```python
from build123d import *

# Parameters (mm, degrees)
SKETCH_1_R               = 15
SKETCH_1_R_2             = 2.3
SKETCH_1_R_3             = 1.1
EXTRUDE_1_DEPTH          = 7
CUT_EXTRUDE_1_DEPTH      = 10
CUT_EXTRUDE_1_DEPTH_BACK = 2
SKETCH_2_R               = 2.1
SKETCH_10_R              = 10
CUT_EXTRUDE_7_DEPTH      = 1.6
SKETCH_9_R               = 4.2
CUT_EXTRUDE_5_DEPTH      = 22.889723616
SKETCH_11_R              = 26.7
SKETCH_11_R_2            = 1.7
EXTRUDE_2_DEPTH          = 5.5
SKETCH_13_R              = 3
CUT_EXTRUDE_9_DEPTH      = 2.5
CUT_EXTRUDE_START        = -8
SKETCH_14_R              = 2.1
CUT_EXTRUDE_10_DEPTH     = 8


with BuildPart() as part:
    # 스케치1 → 보스-돌출1 (new body)
    with BuildSketch(Plane.XY):
        Circle(SKETCH_1_R)
        Circle(SKETCH_1_R_2, mode=Mode.SUBTRACT)
        with Locations((0, 8)):
            Circle(SKETCH_1_R_3, mode=Mode.SUBTRACT)
        with Locations((8, 0)):
            Circle(SKETCH_1_R_3, mode=Mode.SUBTRACT)
        with Locations((0, -8)):
            Circle(SKETCH_1_R_3, mode=Mode.SUBTRACT)
        with Locations((-8, 0)):
            Circle(SKETCH_1_R_3, mode=Mode.SUBTRACT)
    extrude(amount=EXTRUDE_1_DEPTH)

    # 스케치2 → 컷-돌출1 (cut, two sides: drawn at the far end of the back side and taken through both)
    with BuildSketch(Plane.XY.offset(7).offset(-CUT_EXTRUDE_1_DEPTH_BACK)):
        with Locations((0, 8)):
            Circle(SKETCH_2_R)
        with Locations((8, 0)):
            Circle(SKETCH_2_R)
        with Locations((0, -8)):
            Circle(SKETCH_2_R)
        with Locations((-8, 0)):
            Circle(SKETCH_2_R)
    extrude(amount=CUT_EXTRUDE_1_DEPTH + CUT_EXTRUDE_1_DEPTH_BACK, mode=Mode.SUBTRACT)

    # 스케치10 → 컷-돌출7 (cut)
    with BuildSketch(Plane(origin=(0, 0, 0), x_dir=(-1, 0, 0), z_dir=(0, 0, -1))):
        Circle(SKETCH_10_R)
    extrude(amount=-CUT_EXTRUDE_7_DEPTH, mode=Mode.SUBTRACT)

    # 스케치9 → 컷-돌출5 (cut, through all)
    with BuildSketch(Plane(origin=(0, 0, 1.6), x_dir=(-1, 0, 0), z_dir=(0, 0, -1))):
        Circle(SKETCH_9_R)
    extrude(amount=-CUT_EXTRUDE_5_DEPTH, mode=Mode.SUBTRACT)

    # 스케치11 → 보스-돌출2 (add)
    with BuildSketch(Plane.XY.offset(7)):
        Circle(SKETCH_11_R)
        with Locations((-11.254716834, 16.073401413)):
            Circle(SKETCH_11_R_2, mode=Mode.SUBTRACT)
        with Locations((-16.073401413, 11.254716834)):
            Circle(SKETCH_11_R_2, mode=Mode.SUBTRACT)
        with Locations((19.547332366, 1.710169984)):
            Circle(SKETCH_11_R_2, mode=Mode.SUBTRACT)
        with Locations((17.783571397, 8.292615532)):
            Circle(SKETCH_11_R_2, mode=Mode.SUBTRACT)
        with Locations((-8.292615532, -17.783571397)):
            Circle(SKETCH_11_R_2, mode=Mode.SUBTRACT)
        with Locations((-1.710169984, -19.547332366)):
            Circle(SKETCH_11_R_2, mode=Mode.SUBTRACT)
    extrude(amount=EXTRUDE_2_DEPTH)

    # 스케치13 → 컷-돌출9 (cut)
    with BuildSketch(Plane(origin=(0, 0, 7), x_dir=(-1, 0, 0), z_dir=(0, 0, -1))):
        with Locations((-17.783571397, 8.292615532)):
            Circle(SKETCH_13_R)
        with Locations((-19.547332366, 1.710169984)):
            Circle(SKETCH_13_R)
        with Locations((11.254716834, 16.073401413)):
            Circle(SKETCH_13_R)
        with Locations((16.073401413, 11.254716834)):
            Circle(SKETCH_13_R)
        with Locations((1.710169984, -19.547332366)):
            Circle(SKETCH_13_R)
        with Locations((8.292615532, -17.783571397)):
            Circle(SKETCH_13_R)
    extrude(amount=-CUT_EXTRUDE_9_DEPTH, mode=Mode.SUBTRACT)

    # 스케치14 → 컷-돌출10 (cut)
    with BuildSketch(Plane(origin=(0, 0, 7), x_dir=(-1, 0, 0), z_dir=(0, 0, -1)).offset(CUT_EXTRUDE_START)):
        with Locations(Location((8, 0, 0), (0, 0, 180))):
            Circle(SKETCH_14_R)
        with Locations(Location((0, -8, 0), (0, 0, 180))):
            Circle(SKETCH_14_R)
        with Locations(Location((-8, 0, 0), (0, 0, 180))):
            Circle(SKETCH_14_R)
        with Locations(Location((0, 8, 0), (0, 0, 180))):
            Circle(SKETCH_14_R)
    extrude(amount=CUT_EXTRUDE_10_DEPTH, mode=Mode.SUBTRACT)


solid = part.part
```
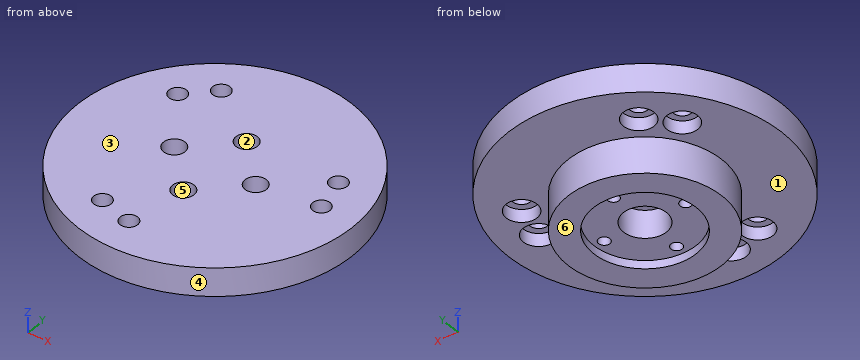
Can you work these out from the model? Positions are in its coordinate system, mm. Face numbers are marked on the shaded views. A direction names the side the tool comes from. Give positions to 0.01 mm unless a question says otherwise; leave off trailing zeros. Loops run counter-clockwise (first coordinate to the right, second up) from the corner with the lowest first, then second, coordinate; pieces in that order, holes last. Notation, with made-up numbers: M 36,-18.75 L 89,-18.75 A7 ccw 89,-10.75 Z; hole C 75,2 d4. An arc over 180 degrees is marked long. Use one line per item in the form item = value. Start each with the question number.
(1) I want a section at B-B, the plane y = -8. Write out the boundary of the cut face in (x, z), and give its area (3 significant figures).
(2) I want a section at C-C, the plane z = 6. Write out the boundary of the cut face in (x, y).
(3) On a 3-axis mill with a long thin cutter (end or side, diameter ignored), from which of +Z, -Z, +X, -X, +Y, -Y can I reach the whole of each face in a straight line? I mean the marked faces 1, 2 and 3. Say none if no direction works.
(4) Please list where these lines run through material, in increasing order: line 1 (Y direction, x = 0, z = 3.1); line 2 (X direction, y = 1, z = 9.25); line 3 (Y direction, x = 0, z = 0.65).
(5) I want a section at D-D, the plane x = 12. Write out the boundary of the cut face in (y, z), and give its area (3 significant figures).
(6) Thinking about a two-plate mould opening in Y: for the marked faces 4, 5 and 6, which applies, released by +Y, released by -Y, zero draft, split by the parting line, or undercut?
(7) I'm going to push flat-ended pins straight in: P1, Ø5, axis at x = -3, y = -18.5, coming from the -Z side; P2, Ø3, axis at x = -16.5, y = 12.5, coming from the -Z side; P3, Ø1.5, axis at x = -14.5, z = 4.5, coming from the +Y side; P4, Ø3.5, axis at x = -0.5, y = -8.5, coming from the +Z side. Where does each tip first touch, or does it pass through?
(8) I want a section at A-A, the plane x = -16.5. Write out the boundary of the cut face in (y, z).
Worked out:
q1.outline = M -25.47,7 L -12.69,7 L -12.69,0 L -6,0 L -6,1.6 L -1.1,1.6 L -1.1,5 L -2.1,5 L -2.1,12.5 L -25.47,12.5 Z; M 1.1,1.6 L 6,1.6 L 6,0 L 12.69,0 L 12.69,7 L 25.47,7 L 25.47,12.5 L 2.1,12.5 L 2.1,5 L 1.1,5 Z
q1.area = 400 mm²
q2.outline = C 0,0 d30; hole C -8,0 d4.2; hole C 0,0 d8.4; hole C 0,-8 d4.2; hole C 0,8 d4.2; hole C 8,0 d4.2
q3.face_1 = -Z
q3.face_2 = +Z
q3.face_3 = +Z, +X, -X, +Y, -Y
q4.line_1 = -15 to -9.1, -6.9 to -4.2, 4.2 to 6.9, 9.1 to 15
q4.line_2 = -26.68 to -9.85, -6.15 to 6.15, 9.85 to 16.63, 22.46 to 26.68
q4.line_3 = -15 to -10, 10 to 15
q5.outline = M -23.85,7 L -9,7 L -9,0 L 9,0 L 9,7 L 23.85,7 L 23.85,12.5 L -23.85,12.5 Z
q5.area = 388 mm²
q6.face_4 = split by the parting line
q6.face_5 = undercut
q6.face_6 = zero draft
q7.P1 = 7
q7.P2 = 9.5
q7.P3 = 5.99
q7.P4 = 12.5
q8.outline = M -20.99,7 L 8.29,7 L 8.29,9.5 L 9.61,9.5 L 9.61,12.5 L -20.99,12.5 Z; M 12.9,9.5 L 14.22,9.5 L 14.22,7 L 20.99,7 L 20.99,12.5 L 12.9,12.5 Z
